Check sheet for the modelled part. Datum: model origin and axes. Units: mm. A direction names the side the tool comes from. Round coordinates to 2 decimals unless told otherwise and drop trailing zeros. Order: outer loops, then holes, each group sorted by start corner. A loop starts at its lowest first (then second) coordinate and runs counter-clockwise, first axis right, second up. Notation, with made-up numbers: (57, 73) -> (64, 73) arc R33 cw to (64, 112) -> close; hole circle Ø7 at (89, -23). An arc over 180 degrees is marked (long way). Answer in a Markdown table with one row per item.
from build123d import *

# Parameters (mm, degrees)
SKIZZE1_W                       = 120
SKIZZE1_H                       = 110
AUFSATZ_LINEAR_AUSTRAGEN1_DEPTH = 2
SKIZZE2_W                       = 4
SKIZZE2_H                       = 85
AUFSATZ_LINEAR_AUSTRAGEN2_DEPTH = 5
SKIZZE3_W                       = 1
SKIZZE3_H                       = 75
AUFSATZ_LINEAR_AUSTRAGEN3_DEPTH = 0.8
SKIZZE4_W                       = 1
SKIZZE4_H                       = 75
AUFSATZ_LINEAR_AUSTRAGEN4_DEPTH = 0.8


with BuildPart() as part:
    # Skizze1 → Aufsatz-Linear austragen1 (new body)
    with BuildSketch(Plane.XY):
        with Locations((2.366105943, 1.130520765)):
            Rectangle(SKIZZE1_W, SKIZZE1_H)
    extrude(amount=AUFSATZ_LINEAR_AUSTRAGEN1_DEPTH)

    # Skizze2 → Aufsatz-Linear austragen2 (add)
    with BuildSketch(Plane.XY.offset(2)):
        with Locations((-51.333894057, 11.230520765)):
            Rectangle(SKIZZE2_W, SKIZZE2_H)
        with Locations((56.066105943, 11.230520765)):
            Rectangle(SKIZZE2_W, SKIZZE2_H)
    extrude(amount=AUFSATZ_LINEAR_AUSTRAGEN2_DEPTH)

    # Skizze3 → Aufsatz-Linear austragen3 (add)
    with BuildSketch(Plane(origin=(58.066105943, 0, 0), x_dir=(0, 0, -1), z_dir=(1, 0, 0))):
        with Locations((-6, 11.230520765)):
            Rectangle(SKIZZE3_W, SKIZZE3_H)
    extrude(amount=AUFSATZ_LINEAR_AUSTRAGEN3_DEPTH)

    # Skizze4 → Aufsatz-Linear austragen4 (add)
    with BuildSketch(Plane.ZY.offset(53.333894057)):
        with Locations((6, 11.230520765)):
            Rectangle(SKIZZE4_W, SKIZZE4_H)
    extrude(amount=AUFSATZ_LINEAR_AUSTRAGEN4_DEPTH)


solid = part.part
Item 1: Scan lines: line 1 (X direction, y = 39, z = 4.25); line 2 (X direction, y = -3.5, z = 6.25); line 3 (Z direction, x = -4.5, y = -34). Record each from-to range of solid material in increasing order. Write a range as [from, to].
Result sheet:
| item | result |
|---|---|
| line 1 | x = [-53.33, -49.33], [54.07, 58.07] |
| line 2 | x = [-54.13, -49.33], [54.07, 58.87] |
| line 3 | z = [0, 2] |
Item 2: Mould release check, pull along X, two halves, no side actions. Record for faces 1 (the flat face through (-51, -31.269, 4)), 2 (the flat face through (54.066, 11, 4)): pulls with the +X half, pulls with the -X half, needs draft (parallel to the pull), parting line crosses it, or undercut.
Result sheet:
| item | result |
|---|---|
| face 1 | needs draft |
| face 2 | undercut |
Item 3: Cross-section at A-A (z = 3.75). Record the boundary of the cut face in (x, y), and give its area (3 significant figures).
Result sheet:
| item | result |
|---|---|
| outline | (-53.33, -31.27) -> (-49.33, -31.27) -> (-49.33, 53.73) -> (-53.33, 53.73) -> close; (54.07, -31.27) -> (58.07, -31.27) -> (58.07, 53.73) -> (54.07, 53.73) -> close |
| area | 680 mm^2 |
Item 4: Set-up check for faces 3 (the flat face through (56, 53.731, 4)), 4 (the flat face through (-51, 12, 7)), 5 (the flat face through (-49.334, 11, 4)), 6 (the flat face through (56, -31.269, 4)), 7 (the flat face through (2, 2, 0)): record each of +Z, -Z, +X, -X, +Y, -Y from which the full face is reachable in a straight line by a thin tool's end or side.
Result sheet:
| item | result |
|---|---|
| face 3 | +Z, +X, -X, +Y |
| face 4 | +Z, +X, -X, +Y, -Y |
| face 5 | +Z, +Y, -Y |
| face 6 | +Z, +X, -X, -Y |
| face 7 | -Z, +X, -X, +Y, -Y |
Item 5: Cross-section at C-C (x = 18.5). Record the boundary of the cut face in (y, z), and give its area (3 significant figures).
Result sheet:
| item | result |
|---|---|
| outline | (-53.87, 0) -> (56.13, 0) -> (56.13, 2) -> (-53.87, 2) -> close |
| area | 220 mm^2 |
Item 6: Cross-section at B-B (y = -7.5). Record the boundary of the cut face in (x, z), and give its area (3 significant figures).
Result sheet:
| item | result |
|---|---|
| outline | (-57.63, 0) -> (62.37, 0) -> (62.37, 2) -> (58.07, 2) -> (58.07, 5.5) -> (58.87, 5.5) -> (58.87, 6.5) -> (58.07, 6.5) -> (58.07, 7) -> (54.07, 7) -> (54.07, 2) -> (-49.33, 2) -> (-49.33, 7) -> (-53.33, 7) -> (-53.33, 6.5) -> (-54.13, 6.5) -> (-54.13, 5.5) -> (-53.33, 5.5) -> (-53.33, 2) -> (-57.63, 2) -> close |
| area | 282 mm^2 |
Item 7: Depth check by flat-ended pin: P1, Ø0.9, axis at x = -54, y = 18, coming from the +Z side; P2, Ø1.5, axis at y = 6, z = 5.5, coming from the -X side; P3, Ø1.2, axis at x = 57, z = 4, coming from the +Y side. Enter the tip coordinate at first touch or a pass-through.
Result sheet:
| item | result |
|---|---|
| P1 | stops at z = 6.5 |
| P2 | stops at x = -54.13 |
| P3 | stops at y = 53.73 |
